Input: part model. Units: mm. Frame: model coordinates. Coordinates: 2 decimals unless noted, no trailing zeros. Order: outer loops, then holes, each group sorted by start corner. A loop starts at its lowest first (then second) coordinate and runs counter-clockwise, first axis right, second up. Notation, with made-up numbers: M -22,-26.5 L 23,-26.5 A20 cw 23,1.5 Z; hole C -3,-35 d8. An arc over 180 degrees is marked long. Answer in a Markdown table with one row per item.
from build123d import *

# Parameters (mm, degrees)
SKETCH_1_W          = 40
SKETCH_1_H          = 160
EXTRUDE_2_DEPTH     = 6
CUT_EXTRUDE_3_DEPTH = 10
SKETCH_5_W          = 40
SKETCH_5_H          = 15
CUT_EXTRUDE_4_DEPTH = 10
CUT_EXTRUDE_5_DEPTH = 10
CUT_EXTRUDE_6_DEPTH = 2
FILLET_1_R          = 1
SKETCH_10_W         = 10
SKETCH_10_H         = 60
EXTRUDE_3_DEPTH     = 4
SKETCH_11_W         = 6
SKETCH_11_H         = 60
CUT_EXTRUDE_7_DEPTH = 4
SKETCH_13_W         = 6
SKETCH_13_H         = 29
EXTRUDE_9_DEPTH     = 2


with BuildPart() as part:
    # Эскиз1 → Бобышка-Вытянуть2 (new body)
    with BuildSketch(Plane.XY):
        Rectangle(SKETCH_1_W, SKETCH_1_H)
    extrude(amount=EXTRUDE_2_DEPTH)

    # Эскиз3 → Вырез-Вытянуть3 (cut)
    with BuildSketch(Plane.XY.offset(6)):
        with BuildLine():
            Line((-3, 55), (-3, 10))
            ThreePointArc((-3, 10), (0, 7), (3, 10))
            Line((3, 10), (3, 55))
            ThreePointArc((3, 55), (0, 58), (-3, 55))
        make_face()
    extrude(amount=-CUT_EXTRUDE_3_DEPTH, mode=Mode.SUBTRACT)

    # Эскиз5 → Вырез-Вытянуть4 (cut)
    with BuildSketch(Plane.XY.offset(6)):
        with Locations((0, 72.5)):
            Rectangle(SKETCH_5_W, SKETCH_5_H)
    extrude(amount=-CUT_EXTRUDE_4_DEPTH, mode=Mode.SUBTRACT)

    # Эскиз7 → Вырез-Вытянуть5 (cut)
    with BuildSketch(Plane.XY.offset(6)):
        with BuildLine():
            Line((-10, -30), (-10, -75))
            ThreePointArc((-10, -75), (-8, -77), (-6, -75))
            Line((-6, -75), (-6, -30))
            ThreePointArc((-6, -30), (-8, -28), (-10, -30))
        make_face()
        with BuildLine():
            Line((-2, -75), (-2, -30))
            ThreePointArc((-2, -30), (0, -28), (2, -30))
            Line((2, -30), (2, -75))
            ThreePointArc((2, -75), (0, -77), (-2, -75))
        make_face()
        with BuildLine():
            Line((6, -75), (6, -30))
            ThreePointArc((6, -30), (8, -28), (10, -30))
            Line((10, -30), (10, -75))
            ThreePointArc((10, -75), (8, -77), (6, -75))
        make_face()
    extrude(amount=-CUT_EXTRUDE_5_DEPTH, mode=Mode.SUBTRACT)

    # Эскиз8 → Вырез-Вытянуть6 (cut)
    # profile 1 of 3: a face of its own
    with BuildSketch(Plane.XY.offset(6)):
        with BuildLine():
            ThreePointArc((-11.5, -30), (-8, -26.5), (-4.5, -30))
            Line((-4.5, -30), (-4.5, -75))
            ThreePointArc((-4.5, -75), (-8, -78.5), (-11.5, -75))
            Line((-11.5, -75), (-11.5, -30))
        make_face()
        with BuildLine():
            Line((-10, -75), (-10, -30))
            ThreePointArc((-10, -30), (-8, -28), (-6, -30))
            Line((-6, -30), (-6, -75))
            ThreePointArc((-6, -75), (-8, -77), (-10, -75))
        make_face(mode=Mode.SUBTRACT)
    # profile 2 of 3: a face of its own
    with BuildSketch(Plane.XY.offset(6)):
        with BuildLine():
            ThreePointArc((-3.5, -30), (0, -26.5), (3.5, -30))
            Line((3.5, -30), (3.5, -75))
            ThreePointArc((3.5, -75), (0, -78.5), (-3.5, -75))
            Line((-3.5, -75), (-3.5, -30))
        make_face()
        with BuildLine():
            ThreePointArc((2, -75), (0, -77), (-2, -75))
            Line((-2, -75), (-2, -30))
            ThreePointArc((-2, -30), (0, -28), (2, -30))
            Line((2, -30), (2, -75))
        make_face(mode=Mode.SUBTRACT)
    # profile 3 of 3: a face of its own
    with BuildSketch(Plane.XY.offset(6)):
        with BuildLine():
            ThreePointArc((4.5, -30), (8, -26.5), (11.5, -30))
            Line((11.5, -30), (11.5, -75))
            ThreePointArc((11.5, -75), (8, -78.5), (4.5, -75))
            Line((4.5, -75), (4.5, -30))
        make_face()
        with BuildLine():
            Line((6, -75), (6, -30))
            ThreePointArc((6, -30), (8, -28), (10, -30))
            Line((10, -30), (10, -75))
            ThreePointArc((10, -75), (8, -77), (6, -75))
        make_face(mode=Mode.SUBTRACT)
    extrude(amount=-CUT_EXTRUDE_6_DEPTH, mode=Mode.SUBTRACT)

    # Скругление1
    # the kernel refuses this fillet: 1 mm, written as the material it takes off along each edge
    with BuildSketch(Plane(origin=(-8, -30, 6), x_dir=(-1, 0, 0), z_dir=(0, -1, 0))) as fillet_1_piece_1:
        with BuildLine():
            CenterArc((3.5 + FILLET_1_R, FILLET_1_R), FILLET_1_R, 180, 90)
            Line((3.5, FILLET_1_R), (3.5, 0))
            Line((3.5, 0), (3.5 + FILLET_1_R, 0))
        make_face()
    revolve(axis=Axis((-8, -30, 6), (0, 0, -1)), revolution_arc=180, mode=Mode.SUBTRACT)
    with BuildSketch(Plane(origin=(-11.5, -75, 6), x_dir=(-1, 0, 0), z_dir=(0, 1, 0)), Plane(origin=(-4.5, -30, 6), x_dir=(1, 0, 0), z_dir=(0, -1, 0)), Plane(origin=(3.5, -30, 6), x_dir=(1, 0, 0), z_dir=(0, -1, 0)), Plane(origin=(-3.5, -75, 6), x_dir=(-1, 0, 0), z_dir=(0, 1, 0)), Plane(origin=(11.5, -30, 6), x_dir=(1, 0, 0), z_dir=(0, -1, 0)), Plane(origin=(4.5, -75, 6), x_dir=(-1, 0, 0), z_dir=(0, 1, 0))) as fillet_1_piece_2:
        with BuildLine():
            CenterArc((FILLET_1_R, -FILLET_1_R), FILLET_1_R, 90, 90)
            Line((0, -FILLET_1_R), (0, 0))
            Line((0, 0), (FILLET_1_R, 0))
        make_face()
    extrude(amount=45, mode=Mode.SUBTRACT)
    with BuildSketch(Plane(origin=(-8, -75, 6), x_dir=(1, 0, 0), z_dir=(0, 1, 0))) as fillet_1_piece_3:
        with BuildLine():
            CenterArc((3.5 + FILLET_1_R, FILLET_1_R), FILLET_1_R, 180, 90)
            Line((3.5, FILLET_1_R), (3.5, 0))
            Line((3.5, 0), (3.5 + FILLET_1_R, 0))
        make_face()
    revolve(axis=Axis((-8, -75, 6), (0, 0, -1)), revolution_arc=180, mode=Mode.SUBTRACT)
    with BuildSketch(Plane(origin=(0, -30, 6), x_dir=(-1, 0, 0), z_dir=(0, -1, 0))) as fillet_1_piece_4:
        with BuildLine():
            CenterArc((3.5 + FILLET_1_R, FILLET_1_R), FILLET_1_R, 180, 90)
            Line((3.5, FILLET_1_R), (3.5, 0))
            Line((3.5, 0), (3.5 + FILLET_1_R, 0))
        make_face()
    revolve(axis=Axis((0, -30, 6), (0, 0, -1)), revolution_arc=180, mode=Mode.SUBTRACT)
    with BuildSketch(Plane(origin=(0, -75, 6), x_dir=(1, 0, 0), z_dir=(0, 1, 0))) as fillet_1_piece_5:
        with BuildLine():
            CenterArc((3.5 + FILLET_1_R, FILLET_1_R), FILLET_1_R, 180, 90)
            Line((3.5, FILLET_1_R), (3.5, 0))
            Line((3.5, 0), (3.5 + FILLET_1_R, 0))
        make_face()
    revolve(axis=Axis((0, -75, 6), (0, 0, -1)), revolution_arc=180, mode=Mode.SUBTRACT)
    with BuildSketch(Plane(origin=(8, -30, 6), x_dir=(-1, 0, 0), z_dir=(0, -1, 0))) as fillet_1_piece_6:
        with BuildLine():
            CenterArc((3.5 + FILLET_1_R, FILLET_1_R), FILLET_1_R, 180, 90)
            Line((3.5, FILLET_1_R), (3.5, 0))
            Line((3.5, 0), (3.5 + FILLET_1_R, 0))
        make_face()
    revolve(axis=Axis((8, -30, 6), (0, 0, -1)), revolution_arc=180, mode=Mode.SUBTRACT)
    with BuildSketch(Plane(origin=(8, -75, 6), x_dir=(1, 0, 0), z_dir=(0, 1, 0))) as fillet_1_piece_7:
        with BuildLine():
            CenterArc((3.5 + FILLET_1_R, FILLET_1_R), FILLET_1_R, 180, 90)
            Line((3.5, FILLET_1_R), (3.5, 0))
            Line((3.5, 0), (3.5 + FILLET_1_R, 0))
        make_face()
    revolve(axis=Axis((8, -75, 6), (0, 0, -1)), revolution_arc=180, mode=Mode.SUBTRACT)

    # Эскиз10 → Бобышка-Вытянуть3 (add)
    with BuildSketch(Plane(origin=(0, 0, 0), x_dir=(-1, 0, 0), z_dir=(0, 0, -1))):
        with Locations((15, 35)):
            Rectangle(SKETCH_10_W, SKETCH_10_H)
    extrude(amount=EXTRUDE_3_DEPTH)

    # Эскиз11 → Вырез-Вытянуть7 (cut)
    with BuildSketch(Plane(origin=(0, 0, -4), x_dir=(-1, 0, 0), z_dir=(0, 0, -1))):
        with Locations((15, 35)):
            Rectangle(SKETCH_11_W, SKETCH_11_H)
    extrude(amount=-CUT_EXTRUDE_7_DEPTH, mode=Mode.SUBTRACT)

    # Эскиз13 → Бобышка-Вытянуть9 (add)
    with BuildSketch(Plane(origin=(0, 0, -4), x_dir=(-1, 0, 0), z_dir=(0, 0, -1))):
        with Locations((17, 50.5)):
            Rectangle(SKETCH_13_W, SKETCH_13_H)
        with Locations((13, 19.5)):
            Rectangle(SKETCH_13_W, SKETCH_13_H)
    extrude(amount=EXTRUDE_9_DEPTH)


solid = part.part
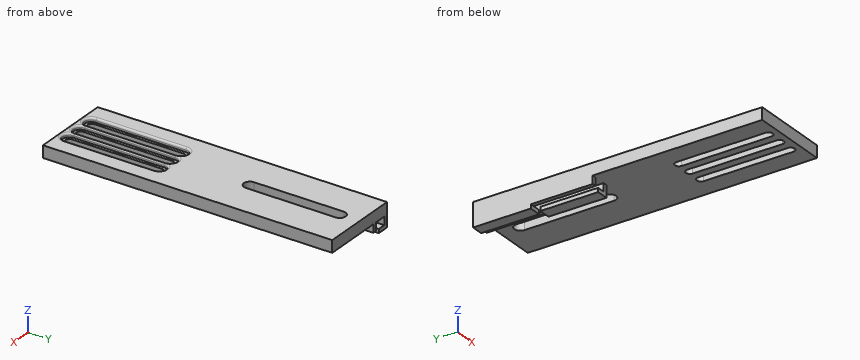
1) Cut plane A-A, the plane x = -8. Output: boundary loops of the cut face in (y, z), and give its area (3 significant figures).
Resolved:
| item | result |
|---|---|
| outline | M -80,0 L -77,0 L -77,4 L -78.5,4 L -78.5,5 A1 ccw -79.5,6 L -80,6 Z; M -28,0 L 65,0 L 65,6 L -25.5,6 A1 ccw -26.5,5 L -26.5,4 L -28,4 Z |
| area | 570 mm2 |
2) Cut plane C-C, the plane z = 2. Output: boundary loops of the cut face in (x, y), and give its area (3 significant figures).
Resolved:
| item | result |
|---|---|
| outline | M -20,-80 L 20,-80 L 20,65 L -20,65 Z; hole M -10,-75 A2 ccw -6,-75 L -6,-30 A2 ccw -10,-30 Z; hole M -3,10 A3 ccw 3,10 L 3,55 A3 ccw -3,55 Z; hole M -2,-75 A2 ccw 2,-75 L 2,-30 A2 ccw -2,-30 Z; hole M 6,-75 A2 ccw 10,-75 L 10,-30 A2 ccw 6,-30 Z |
| area | 4,920 mm2 |
3) Material intervals for probe 1 along X at (y, z) = (-71.5, 3.5); probe 2 along Y at (x, z) = (0, 0.5); probe 3 along X at (y, z) = (20.5, 3.25), sorted ascending.
Resolved:
| item | result |
|---|---|
| probe 1 | x = -20 to -10, -6 to -2, 2 to 6, 10 to 20 |
| probe 2 | y = -80 to -77, -28 to 7, 58 to 65 |
| probe 3 | x = -20 to -3, 3 to 20 |
4) Cut plane B-B, the plane y = 50. Output: boundary loops of the cut face in (x, z), and give its area (3 significant figures).
Resolved:
| item | result |
|---|---|
| outline | M -20,-6 L -14,-6 L -14,-4 L -18,-4 L -18,0 L -12,0 L -12,-4 L -10,-4 L -10,0 L -3,0 L -3,6 L -20,6 Z; M 3,0 L 20,0 L 20,6 L 3,6 Z |
| area | 232 mm2 |
5) Contact query for flat-ended pins moving along their axis: pin 1 (2 mm diameter, centred on x = -12, z = -5.5, fed in from +Y); pin 2 (0.6 mm diameter, centred on x = -19.5, y = 26.5, fed in from -Z); pin 3 (2 mm diameter, centred on x = -16.5, z = -4.5, fed in from -Y). Output: stop coordinate, or through.
Resolved:
| item | result |
|---|---|
| pin 1 | stops at y = 34 |
| pin 2 | stops at z = -4 |
| pin 3 | stops at y = 5 |
6) Cut plane D-D, the plane x = 0. Output: boundary loops of the cut face in (y, z), and give its area (3 significant figures).
Resolved:
| item | result |
|---|---|
| outline | M -80,0 L -77,0 L -77,4 L -78.5,4 L -78.5,5 A1 ccw -79.5,6 L -80,6 Z; M -28,0 L 7,0 L 7,6 L -25.5,6 A1 ccw -26.5,5 L -26.5,4 L -28,4 Z; M 58,0 L 65,0 L 65,6 L 58,6 Z |
| area | 264 mm2 |
